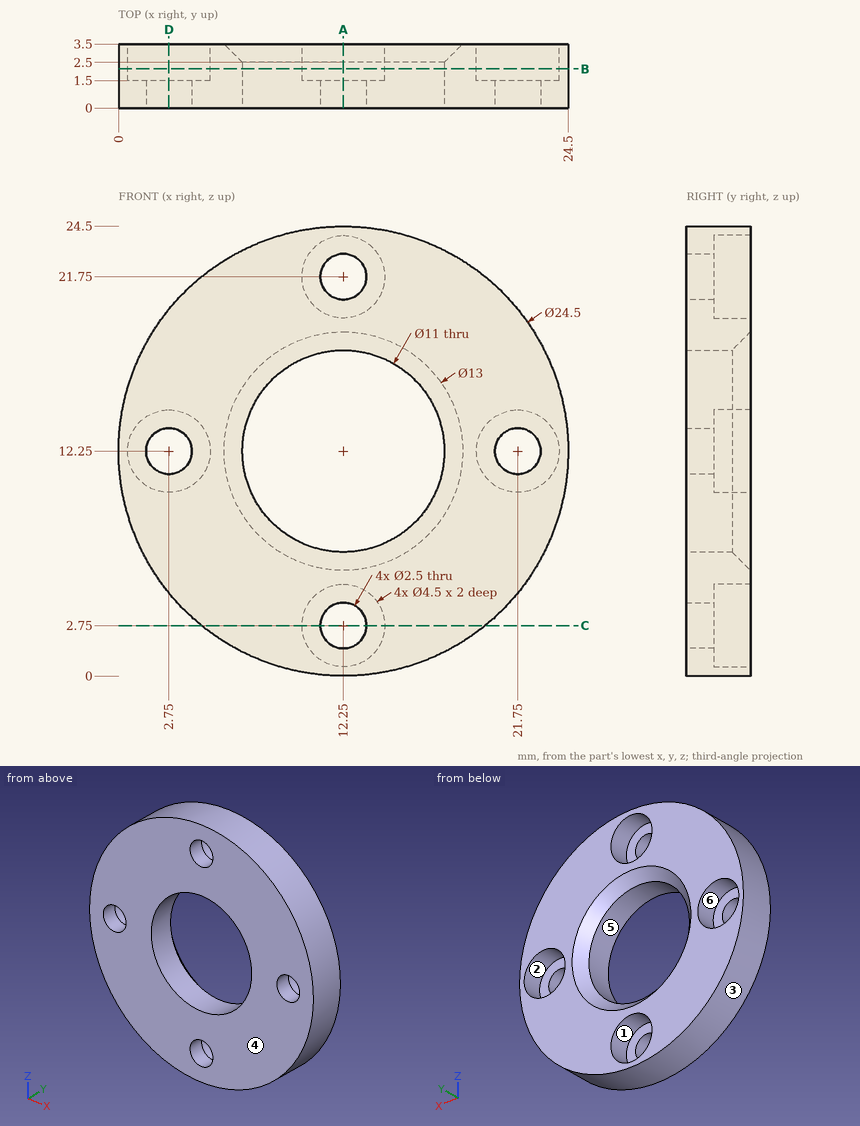
Check sheet for the drawn part. Datum: minimum x, y, z corner. Units: mm. A direction names the side the tool comes from. Coordinates: 2 decimals unless noted, no trailing zeros. Order: outer loops, then holes, each group sorted by start corner. A loop starts at its lowest first (then second) coordinate and runs counter-clockwise, first axis right, second up. Notation, with made-up numbers: (-18.5, 64.25) -> (-7.5, 64.25) arc R29 ccw to (-7.5, 103.25) -> close; hole circle Ø2 at (59, 79.25). An arc over 180 degrees is marked (long way). Use a Markdown table: item, result. Add a question column.
1. Go/stop test with flat-tipped pins: pin 1 Ø2 at (x, z) = (12.5, 3) entering from +Y; pin 2 Ø2 at (y, z) = (3, 9.5) entering from -X. Record where each tip stops, or that it passes through.
2. Material ranges on L1, parallel to X at y = 1.15, z = 12.25; L2, parallel to Z at x = 11, y = 1.9; L3, parallel to X at y = 2.8, z = 12.25, recorded low to high.
3. Cross-section at A-A (x = 12.25). Enter the section's corners in (y, z).
4. Cross-section at B-B (y = 2.15). Enter the section's corners in (x, z).
5. Cross-section at D-D (x = 2.75). Enter the section's corners in (y, z).
6. Cross-section at C-C (z = 2.75). Enter the section's corners in (x, y), and give its area (3 significant figures).
7. Mould release check, pull along Z, two halves, no side actions. Record for the marked faces 1, 2, 3 and 4: pulls with the +Z half, pulls with the -Z half, needs draft (parallel to the pull), parting line crosses it, or undercut.
8. Set-up check for the marked faces 5 and 6: record each of +Z, -Z, +X, -X, +Y, -Y from which the full face is reachable in a straight line by a thin tool's end or side.
Filled sheet:
| question | item | result |
|---|---|---|
| 1 | pin 1 | y = 1.5 |
| 1 | pin 2 | x = 0.13 |
| 2 | L1 | 0 to 1.5, 4 to 6.75, 17.75 to 20.5, 23 to 24.5 |
| 2 | L2 | 0.06 to 0.88, 4.62 to 6.89, 17.61 to 19.88, 23.62 to 24.44 |
| 2 | L3 | 0 to 0.5, 5 to 6.45, 18.05 to 19.5, 24 to 24.5 |
| 3 | outline | (0, 0) -> (3.5, 0) -> (3.5, 0.5) -> (1.5, 0.5) -> (1.5, 1.5) -> (0, 1.5) -> close; (0, 4) -> (1.5, 4) -> (1.5, 5) -> (3.5, 5) -> (3.5, 5.75) -> (2.5, 6.75) -> (0, 6.75) -> close; (0, 17.75) -> (2.5, 17.75) -> (3.5, 18.75) -> (3.5, 19.5) -> (1.5, 19.5) -> (1.5, 20.5) -> (0, 20.5) -> close; (0, 23) -> (1.5, 23) -> (1.5, 24) -> (3.5, 24) -> (3.5, 24.5) -> (0, 24.5) -> close |
| 4 | outline | circle Ø24.5 at (12.25, 12.25); hole circle Ø4.5 at (2.75, 12.25); hole circle Ø11 at (12.25, 12.25); hole circle Ø4.5 at (12.25, 2.75); hole circle Ø4.5 at (12.25, 21.75); hole circle Ø4.5 at (21.75, 12.25) |
| 5 | outline | (0, 4.52) -> (3.5, 4.52) -> (3.5, 10) -> (1.5, 10) -> (1.5, 11) -> (0, 11) -> close; (0, 13.5) -> (1.5, 13.5) -> (1.5, 14.5) -> (3.5, 14.5) -> (3.5, 19.98) -> (0, 19.98) -> close |
| 6 | outline | (4.52, 0) -> (11, 0) -> (11, 1.5) -> (10, 1.5) -> (10, 3.5) -> (4.52, 3.5) -> close; (13.5, 0) -> (19.98, 0) -> (19.98, 3.5) -> (14.5, 3.5) -> (14.5, 1.5) -> (13.5, 1.5) -> close |
| 6 | area | 41.4 mm2 |
| 7 | face 1 | undercut |
| 7 | face 2 | undercut |
| 7 | face 3 | parting line crosses it |
| 7 | face 4 | needs draft |
| 8 | face 5 | +Y, -Y |
| 8 | face 6 | +Y |
